from build123d import *

# Parameters (mm, degrees)
PAD_DEPTH       = 13.79
PAD001_DEPTH    = 48.7
PAD002_DEPTH    = 46.8
SKETCH002_W     = 31.2
SKETCH002_H     = 10
POCKET_DEPTH    = 14
POCKET001_DEPTH = 10
FILLET_R        = 6
SKETCH004_W     = 2
SKETCH004_H     = 11
POCKET002_DEPTH = 10
POCKET003_DEPTH = 10
FILLET001_R     = 2


with BuildPart() as part:
    # Sketch → Pad (new body)
    with BuildSketch(Plane.XZ):
        Polygon((34.35, 0), (-34.35, 0), (-37.9, -3.5), (-41.2, -18), (41.2, -18), (37.9, -3.5), align=None)
    extrude(amount=PAD_DEPTH)

    # Sketch → Pad001 (join)
    with BuildSketch(Plane.XZ):
        Polygon((34.35, 0), (-34.35, 0), (-37.9, -3.5), (-41.2, -18), (41.2, -18), (37.9, -3.5), align=None)
    extrude(amount=-PAD001_DEPTH)

    # Sketch001 → Pad002 (join)
    with BuildSketch(Plane.XZ):
        Polygon((-18.95, 0), (-18.95, 5.83), (-23.1, 5.83), (-23.1, 10), (23.1, 10), (23.1, 5.83), (18.95, 5.83), (18.95, 0), align=None)
    extrude(amount=-PAD002_DEPTH)

    # Sketch002 → Pocket (cut)
    with BuildSketch(Plane.XZ):
        with Locations((0, 5)):
            Rectangle(SKETCH002_W, SKETCH002_H)
    extrude(amount=-POCKET_DEPTH, mode=Mode.SUBTRACT)

    # Sketch003 → Pocket001 (cut)
    with BuildSketch(Plane.XY):
        Polygon((18.1, 0), (23.1, 8), (23.1, 0), align=None)
        Polygon((-23.1, 0), (-23.1, 8), (-18.1, 0), align=None)
    extrude(amount=POCKET001_DEPTH, mode=Mode.SUBTRACT)

    # Fillet
    fillet_edges = [part.edges().sort_by_distance(p)[0] for p in [
        (39.55, -13.79, -10.75),
        (-39.55, -13.79, -10.75),
    ]]
    fillet(fillet_edges, radius=FILLET_R)

    # Sketch004 → Pocket002 (cut)
    with BuildSketch(Plane.XY):
        with Locations((-12, 19.5)):
            Rectangle(SKETCH004_W, SKETCH004_H)
        with Locations((-4, 19.5)):
            Rectangle(SKETCH004_W, SKETCH004_H)
        with Locations((4, 19.5)):
            Rectangle(SKETCH004_W, SKETCH004_H)
        with Locations((12, 19.5)):
            Rectangle(SKETCH004_W, SKETCH004_H)
    extrude(amount=POCKET002_DEPTH, mode=Mode.SUBTRACT)

    # Sketch005 (on Face25 of Pocket002) → Pocket003 (cut)
    with BuildSketch(Plane(origin=(0, 0, 10), x_dir=(-1, 0, 0), z_dir=(0, 0, 1))):
        Polygon((13, -15), (14, -14), (13, -14), align=None)
        Polygon((11, -14), (11, -15), (10, -14), align=None)
        Polygon((5, -15), (6, -14), (5, -14), align=None)
        Polygon((2, -14), (3, -15), (3, -14), align=None)
        Polygon((-3, -14), (-3, -15), (-2, -14), align=None)
        Polygon((-6, -14), (-5, -15), (-5, -14), align=None)
        Polygon((-11, -14), (-11, -15), (-10, -14), align=None)
        Polygon((-13, -14), (-13, -15), (-14, -14), align=None)
    extrude(amount=-POCKET003_DEPTH, mode=Mode.SUBTRACT)

    # Fillet001
    fillet001_edges = [part.edges().sort_by_distance(p)[0] for p in [
        (23.1, 8, 7.915),
        (-23.1, 8, 7.915),
    ]]
    fillet(fillet001_edges, radius=FILLET001_R)


solid = part.part
For this review, take the finished solid that the model builds, in its own axes (mm). A direction names the side the tool comes from. Round coordinates to 2 decimals unless told otherwise and drop trailing zeros. Order: outer loops, then holes, each group sorted by start corner. A loop starts at its lowest first (then second) coordinate and runs counter-clockwise, first axis right, second up. Notation, with made-up numbers: M 36,-26 L 67,-26 A21 ccw 67,6 Z; hole C 41,2.5 d2. An arc over 180 degrees is marked long. Use a Markdown table: item, result. Add a question column.
Item 1: Insertion check: pin 1 (3 mm diameter, centred on y = 18.5, z = 4.5, fed in from +X); pin 2 (0.6 mm diameter, centred on x = -12, z = 6, fed in from -Y); pin 3 (11 mm diameter, centred on y = 19.5, z = 4.5, fed in from -X). Each pin has a flat end and moves straight along its axis. Give the tip position at first contact, or say it passes through.
Item 2: Mouldability with a two-part tool opening along X and no side actions: class faces 1 (the flat face through (-19.959, 2.975, 7.152)), 2 (the flat face through (-13, 20, 5)), 3 (the flat face through (19.893, 2.869, 7.152)) as released by +X, released by -X, zero draft, split by the parting line, or undercut.
Item 3: To check wall thickness, follow line 1 along X through (y, z) = (4.5, 1); line 2 along Z through (x, y) = (19.5, 19.5); line 3 along X through (y, z) = (16, 4.5). State the ranges of each line that lie inside material, in increasing order.
Item 4: Add section D-D, the plane y = 30. Give the boundary of the cut face in (x, z), then the cut area to 3 significant figures.
Item 5: Add section C-C, the plane x = 0. Give the boundary of the cut face in (y, z), then the cut area to 3 significant figures.
Item 6: Tool access review of faces 4 (the flat face through (3, 20, 5)), 5 (the flat face through (23.1, 27, 8)), 6 (the flat face through (-21, 24, 5.83)), 7 (the flat face through (0, 46.8, 5)): name each direction out of +Z, -Z, +X, -X, +Y, -Y from which nothing blocks a thin tool from reaching the whole face with its end or side.
Item 7: Add section A-A, the plane x = -21.5. Give the boundary of the cut face in (y, z), then the cut area to 3 significant figures.
Item 8: Add section B-B, the plane y = -6.5. Give the boundary of the cut face in (x, z).
Geometry results:
| question | item | result |
|---|---|---|
| 1 | pin 1 | stops at x = 23.1 |
| 1 | pin 2 | stops at y = 25 |
| 1 | pin 3 | stops at x = -35.36 |
| 2 | face 1 | released by -X |
| 2 | face 2 | undercut |
| 2 | face 3 | released by +X |
| 3 | line 1 | x = -18.95 to -15.6, 15.6 to 18.95 |
| 3 | line 2 | z = -18 to 0, 5.83 to 10 |
| 3 | line 3 | x = -18.95 to -13, -11 to -5, -3 to 3, 5 to 11, 13 to 18.95 |
| 4 | outline | M -41.2,-18 L 41.2,-18 L 37.9,-3.5 L 34.35,0 L 18.95,0 L 18.95,5.83 L 23.1,5.83 L 23.1,10 L -23.1,10 L -23.1,5.83 L -18.95,5.83 L -18.95,0 L -34.35,0 L -37.9,-3.5 Z |
| 4 | area | 1,810 mm² |
| 5 | outline | M -13.79,-18 L 48.7,-18 L 48.7,0 L 46.8,0 L 46.8,10 L 14,10 L 14,0 L -13.79,0 Z |
| 5 | area | 1,450 mm² |
| 6 | face 4 | +Z, -Y |
| 6 | face 5 | +Z, +X, +Y, -Y |
| 6 | face 6 | -X, +Y, -Y |
| 6 | face 7 | +Z, +X, -X, +Y |
| 7 | outline | M -13.79,-18 L 48.7,-18 L 48.7,0 L -13.79,0 Z; M 5.44,5.83 L 46.8,5.83 L 46.8,10 L 5.44,10 Z |
| 7 | area | 1,300 mm² |
| 8 | outline | M -41.2,-18 L 41.2,-18 L 37.9,-3.5 L 34.35,0 L -34.35,0 L -37.9,-3.5 Z |
